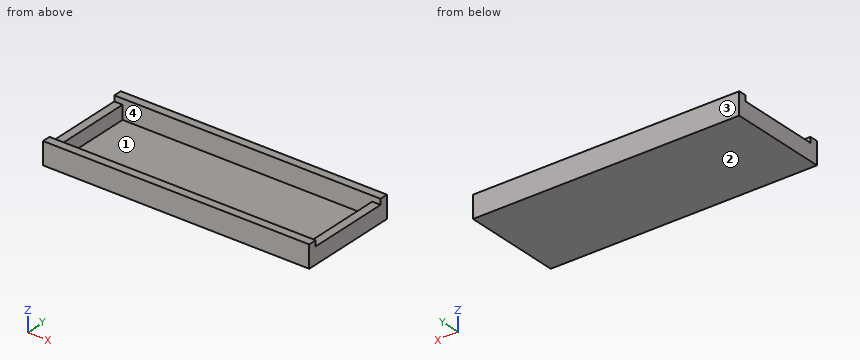
```python
from build123d import *

# Parameters (mm, degrees)
F0_W     = 1219.2
F0_H     = 457.2
F1_DEPTH = 12.7
F2_W     = 1219.2
F2_H     = 38.1
F3_DEPTH = 88.9
F4_W     = 38.1
F4_H     = 381
F5_DEPTH = 63.5


# Not quite as in the source:
# - a length typed as a fraction of an inch, garbled in the dataset ("3 / 203.2 mm" for 3/8 in), is restored


with BuildPart() as f1:
    # F0 (on Top) → F1 (new body)
    with BuildSketch(Plane.XY):
        Rectangle(F0_W, F0_H)
    extrude(amount=F1_DEPTH)

    # F2 (on face) → F3 (join)
    with BuildSketch(Plane.XY.offset(12.7)):
        with Locations((0, -209.55)):
            Rectangle(F2_W, F2_H)
        with Locations((0, 209.55)):
            Rectangle(F2_W, F2_H)
    extrude(amount=F3_DEPTH)

    # F4 (on face) → F5 (join)
    with BuildSketch(Plane.XY.offset(12.7)):
        with Locations((-590.55, 0)):
            Rectangle(F4_W, F4_H)
        with Locations((590.55, 0)):
            Rectangle(F4_W, F4_H)
    extrude(amount=F5_DEPTH)


solid = f1.part
```
Design review of the part built by this model. Coordinates are the model's own, in mm. Face numbers are marked on the shaded views. A direction names the side the tool comes from. Coordinates: 2 decimals unless noted, no trailing zeros. Order: outer loops, then holes, each group sorted by start corner. A loop starts at its lowest first (then second) coordinate and runs counter-clockwise, first axis right, second up. Notation, with made-up numbers: (-29.75, 21) - (-1.75, 21) arc R26 cw to (-1.75, 58) - close; hole circle Ø10 at (56.5, 20.25). An arc over 180 degrees is marked (long way). One line per question, with ' | ' between items.
Q1. To check wall thickness, follow line 1 along Y through (x, z) = (-414, 48.5); line 2 along X through (y, z) = (-142, 67); line 3 along Z through (x, y) = (72.5, 183). State the ranges of each line that lie inside material, in increasing order.
Answer key:
line 1: y = -228.6 to -190.5, 190.5 to 228.6 | line 2: x = -609.6 to -571.5, 571.5 to 609.6 | line 3: z = 0 to 12.7
Q2. Consider section A-A, the plane z = 24.5. Give the boundary of the cut face in (x, y), then the cut area to 3 significant figures.
Answer key:
outline: (-609.6, -228.6) - (609.6, -228.6) - (609.6, 228.6) - (-609.6, 228.6) - close; hole (-571.5, -190.5) - (571.5, -190.5) - (571.5, 190.5) - (-571.5, 190.5) - close | area: 122,000 mm2
Q3. For the marked faces 1 and 2, list the 3-axis set-ups (+Z, -Z, +X, -X, +Y, -Y) from which the entire face can be reached by the end or side of a thin tool; tool diameter is ignored.
Answer key:
face 1: +Z | face 2: -Z, +X, -X, +Y, -Y
Q4. Consider section C-C, the plane y = 102. Give the boundary of the cut face in (x, z), then the cut area to 3 significant figures.
Answer key:
outline: (-609.6, 0) - (609.6, 0) - (609.6, 76.2) - (571.5, 76.2) - (571.5, 12.7) - (-571.5, 12.7) - (-571.5, 76.2) - (-609.6, 76.2) - close | area: 20,300 mm2
Q5. The part is to be moulded in two halves that separate along X. For the marked faces 3 and 4, say which applies: +X half, -X half, draft (parallel to the pull), parting line (faces both ways), or undercut.
Answer key:
face 3: draft | face 4: undercut
Q6. Clearance check with flat-ended pins moving along their axes: pin 1 Ø12 at (x, y) = (31.5, -132.5) entering from -Z; pin 2 Ø6 at (x, y) = (66, -115) entering from +Z; pin 3 Ø11.5 at (x, y) = (-599, 78) entering from +Z. State where each tip first meets the part, or that it passes through.
Answer key:
pin 1: stops at z = 0 | pin 2: stops at z = 12.7 | pin 3: stops at z = 76.2
Q7. Consider section B-B, the plane x = 404. Give the boundary of the cut face in (y, z), then the cut area to 3 significant figures.
Answer key:
outline: (-228.6, 0) - (228.6, 0) - (228.6, 101.6) - (190.5, 101.6) - (190.5, 12.7) - (-190.5, 12.7) - (-190.5, 101.6) - (-228.6, 101.6) - close | area: 12,600 mm2
